from build123d import *

# Parameters (mm, degrees)
BOSS_EXTRUDE1_DEPTH = 6
CUT_EXTRUDE1_DEPTH  = 73.882968029


with BuildPart() as part:
    # Sketch1 → Boss-Extrude1 (new body)
    with BuildSketch(Plane.XY):
        Polygon((28.6385, 47.625), (28.6385, 41.0972), (34.6329, 41.0972), (34.6329, 38.1), (37.8079, 38.1), (37.8079, 41.0972), (40.9829, 41.0972), (40.9829, 35.1028), (28.6385, 35.1028), (28.6385, 15.6972), (40.9829, 15.6972), (40.9829, 9.7028), (37.8079, 9.7028), (37.8079, 12.7), (34.6329, 12.7), (34.6329, 9.7028), (28.6385, 9.7028), (28.6385, 3.175), (15.8115, -47.625), (9.2837, -47.625), (9.2837, -53.6194), (6.2865, -53.6194), (6.2865, -56.7944), (9.2837, -56.7944), (9.2837, -59.9694), (3.2893, -59.9694), (3.2893, -47.625), (-16.1163, -47.625), (-16.1163, -59.9694), (-22.1107, -59.9694), (-22.1107, -56.7944), (-19.1135, -56.7944), (-19.1135, -53.6194), (-22.1107, -53.6194), (-22.1107, -47.625), (-28.6385, -47.625), align=None)
    extrude(amount=BOSS_EXTRUDE1_DEPTH)

    # Sketch2 → Cut-Extrude1 (cut, through all)
    with BuildSketch(Plane.XY.offset(6)):
        Polygon((14.189592964, 6.000975012), (7.84117256, -4.556265128), (12.978303844, -7.645393407), (19.326724249, 2.911846732), align=None)
        Polygon((1.100066357, -15.766530432), (6.237197642, -18.855658711), (-0.111222762, -29.412898851), (-5.248354047, -26.323770571), align=None)
    extrude(amount=-CUT_EXTRUDE1_DEPTH, mode=Mode.SUBTRACT)


solid = part.part
Model file for the job. Use its own axes, mm. A direction names the side the tool comes from. Give positions to 0.01 mm unless a question says otherwise; leave off trailing zeros. Write each loop counter-clockwise with the first axis right and the second up, starting at its lowest first coordinate (ties: lowest second). Pieces come first, ordered by that corner, then holes. Notation, with made-up numbers: M 38,68 L 44,68 A32 cw 44,101 Z; hole C 83,-27.5 d5. An arc over 180 degrees is marked long. One line per item, written item: value. Start each with the question number.
Q1. Saw through at D-D, the plane y = 31.5. Write the cut outline in (x, z), plus the area to 3 significant figures.
Q2. Saw through at A-A, the plane y = -3.5. Write the cut outline in (x, z).
Q3. Probe probe 1 along Y at (x, z) = (31, 0.75); probe 2 along Y at (x, z) = (9, 3.75); probe 3 along X at (y, z) = (10, 0.75). List the from-to ranges inside material, lowest first. Write a range as [from, to].
Q4. Two-plate mould, pull along Y, no slides. Class faces 1 (the flat face through (35, 15.697, 3)), 2 (the flat face through (32, 41.097, 3)), 3 (the flat face through (28.638, 26, 3)), 4 (the flat face through (34.633, 40, 3)): +Y half, -Y half, draft (parallel to the pull), parting line (faces both ways), or undercut.
Q5. Drop flat-ended pins along their axis: pin 1 Ø2.5 at (y, z) = (-58, 2) entering from -X; pin 2 Ø3.5 at (y, z) = (40, 4) entering from -X; pin 3 Ø1.5 at (x, z) = (32, 3.5) entering from +Y. Give the stop position or say it passes through.
Q6. Saw through at B-B, the plane x = -3. Write the cut outline in (y, z) (3 decimals).
Q7. Saw through at C-C, the plane z = 3. State how many separate pieces and enclosed holes the cut face has, plus the area to 3 significant figures.
Q8. 3-axis set-ups, long thin cutter, end or side, ignore diameter. For faces 5 (the flat face through (-2.64, -27.89, 3.04)), 6 (the flat face through (8, -56.794, 3)), 7 (the flat face through (28.638, 6, 3)), 8 (the flat face through (37.808, 11, 3)): which of +Z, -Z, +X, -X, +Y, -Y reach the whole face in a straight line?
Output values:
1. outline: M 18.94,0 L 28.64,0 L 28.64,6 L 18.94,6 Z
1. area: 58.2 mm²
2. outline: M -2.1,0 L 8.48,0 L 8.48,6 L -2.1,6 Z; M 15.47,0 L 26.95,0 L 26.95,6 L 15.47,6 Z
3. probe 1: y = [9.7, 15.7], [35.1, 41.1]
3. probe 2: y = [-59.97, -56.79], [-53.62, -5.25], [-2.63, 14.97]
3. probe 3: x = [6.01, 34.63], [37.81, 40.98]
4. face 1: undercut
4. face 2: +Y half
4. face 3: undercut
4. face 4: draft
5. pin 1: stops at x = -22.11
5. pin 2: stops at x = 23
5. pin 3: stops at y = 41.1
6. outline: M -47.625,0 L -27.676,0 L -27.676,6 L -47.625,6 Z; M -22.585,0 L -4.989,0 L -4.989,6 L -22.585,6 Z
7. separate pieces: 1
7. enclosed holes: 2
7. area: 2,510 mm²
8. face 5: +Z, -Z
8. face 6: +Z, -Z, +X
8. face 7: +Z, -Z, +X, -Y
8. face 8: +Z, -Z, -Y
